Design review of the part built by this model. Coordinates are the model's own, in mm. Face numbers are marked on the shaded views. A direction names the side the tool comes from. Round coordinates to 2 decimals unless told otherwise and drop trailing zeros. Loops run counter-clockwise (first coordinate to the right, second up) from the corner with the lowest first, then second, coordinate; pieces in that order, holes last. Notation, with made-up numbers: M 15,70 L 60,70 A20 ccw 60,76 Z; hole C 41,39.25 d9. An arc over 180 degrees is marked long. Answer as CSV lines item,"result". Start each with the question number.
from build123d import *

# Parameters (mm, degrees)
F0_W      = 54
F0_H      = 56
F1_DEPTH  = 102
F2_W      = 90
F2_H      = 36
F3_DEPTH  = 59.1
F6_DEPTH  = 25
F7_W      = 18
F7_H      = 54
F8_DEPTH  = 8
F9_W      = 24
F9_H      = 54
F10_DEPTH = 8
F11_W     = 36
F11_H     = 54
F12_DEPTH = 8
F14_DEPTH = 12
F16_DEPTH = 25
F18_DEPTH = 42.4
F20_DEPTH = 25


with BuildPart() as f1:
    # F0 (on Right) → F1 (new body)
    with BuildSketch(Plane.YZ):
        with Locations((-4.050715, 4.935318)):
            Rectangle(F0_W, F0_H)
    extrude(amount=F1_DEPTH)

    # F2 (on face) → F3 (cut)
    with BuildSketch(Plane(origin=(0, 22.949285, 0), x_dir=(-1, 0, 0), z_dir=(0, 1, 0))):
        with Locations((-57, -5.064682)):
            Rectangle(F2_W, F2_H)
    extrude(amount=-F3_DEPTH, mode=Mode.SUBTRACT)

    # F5 (on face) → F6 (cut)
    with BuildSketch(Plane(origin=(0, 0, 0), x_dir=(0, -1, 0), z_dir=(-1, 0, 0))):
        Polygon((-2.864712, -16.520232), (11.135288, -16.520232), (20.040549, -5.717624), (11.135288, 5.084983), (-2.864712, 5.084983), (-11.769973, -5.717624), align=None)
    extrude(amount=-F6_DEPTH, mode=Mode.SUBTRACT)

    # F7 (on face) → F8 (cut)
    with BuildSketch(Plane.XY.offset(32.935318)):
        with Locations((9, -4.050715)):
            Rectangle(F7_W, F7_H)
    extrude(amount=-F8_DEPTH, mode=Mode.SUBTRACT)

    # F9 (on face) → F10 (cut)
    with BuildSketch(Plane.XY.offset(32.935318)):
        with Locations((42, -4.050715)):
            Rectangle(F9_W, F9_H)
    extrude(amount=-F10_DEPTH, mode=Mode.SUBTRACT)

    # F11 (on face) → F12 (cut)
    with BuildSketch(Plane.XY.offset(32.935318)):
        with Locations((84, -4.050715)):
            Rectangle(F11_W, F11_H)
    extrude(amount=-F12_DEPTH, mode=Mode.SUBTRACT)

    # F13 (on face) → F14 (cut)
    with BuildSketch(Plane.YZ.offset(66)):
        Polygon((16.72348, 32.935318), (-4.050715, 32.935318), (-4.050715, 24.935318), align=None)
    extrude(amount=-F14_DEPTH, mode=Mode.SUBTRACT)

    # F15 (on face) → F16 (cut)
    with BuildSketch(Plane.YZ.offset(66)):
        Polygon((-4.050715, 32.935318), (-24.917709, 32.935318), (-4.050715, 24.935318), align=None)
    extrude(amount=-F16_DEPTH, mode=Mode.SUBTRACT)

    # F17 (on face) → F18 (cut)
    with BuildSketch(Plane(origin=(0, 0, 0), x_dir=(0, -1, 0), z_dir=(-1, 0, 0))):
        Polygon((26.28649, 33.151057), (-16.84958, 33.434331), (4.061393, 24.936128), align=None)
    extrude(amount=-F18_DEPTH, mode=Mode.SUBTRACT)

    # F19 (on face) → F20 (cut)
    with BuildSketch(Plane.XY.offset(24.935318)):
        Polygon((96, -19.514816), (102, -16.050715), (102, 7.949285), (96, 11.413387), align=None)
    extrude(amount=-F20_DEPTH, mode=Mode.SUBTRACT)


solid = f1.part
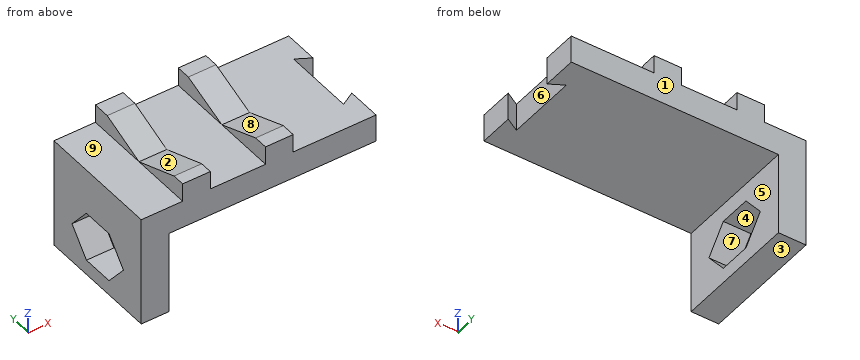
Item 1: Consider section C-C, the plane y = -2. Write out the cut boundary in (x, z), then the cut area to 3 significant figures.
Item 2: Consider section D-D, the plane z = 19. Write out the cut boundary in (x, y).
Item 3: Insertion check: pin 1 Ø14.5 at (x, y) = (8.5, -12.5) entering from +Z; pin 2 Ø6 at (y, z) = (-11.5, 16.5) entering from +X; pin 3 Ø6.5 at (y, z) = (-23, 28) entering from +X; pin 4 Ø4 at (x, y) = (26, 8.5) entering from -Z. Each pin has a flat end and moves straight along its axis. Give the tip position at first contact, or say it passes through.
Item 4: Consider section A-A, the plane z = 2.5. Write out the cut boundary in (x, y).
Item 5: Consider section B-B, the plane x = 28.5. Write out the cut boundary in (y, z).
Item 6: To check wall thickness, follow line 1 (X direction, y = -21, z = 26.5); line 2 (X direction, y = -9, z = 18.5); line 3 (Z direction, x = 10, y = 12.5). State the ranges of each line that lie inside material, in increasing order.
Item 7: The part is to be moulded in two halves that separate along Y. For the marked faces 1, 2, 3 and 4, say which applies: +Y half, -Y half, draft (parallel to the pull), parting line (faces both ways), or undercut.
Item 8: Tool access review of the marked faces 5, 6, 7, 8 and 9: name each direction out of +Z, -Z, +X, -X, +Y, -Y from which nothing blocks a thin tool from reaching the whole face with its end or side.
Found:
1,outline,"M 0,-23.06 L 12,-23.06 L 12,-16.52 L 0,-16.52 Z; M 0,5.08 L 12,5.08 L 12,12.94 L 96,12.94 L 96,24.94 L 66,24.94 L 66,25.73 L 54,25.73 L 54,24.94 L 30,24.94 L 30,25.77 L 18,25.77 L 18,24.94 L 0,24.94 Z"
1,area,"1,340 mm^2"
2,outline,"M 0,-31.05 L 102,-31.05 L 102,-16.05 L 96,-19.51 L 96,11.41 L 102,7.95 L 102,22.95 L 0,22.95 Z"
3,pin 1,"stops at z = 24.94"
3,pin 2,"stops at x = 96"
3,pin 3,"stops at x = 102"
3,pin 4,"stops at z = 12.94"
4,outline,"M 0,-31.05 L 12,-31.05 L 12,-13.27 L 0,-13.27 Z; M 0,5 L 12,5 L 12,22.95 L 0,22.95 Z"
5,outline,"M -31.05,12.94 L 22.95,12.94 L 22.95,32.94 L 15.62,32.94 L -4.06,24.94 L -25.7,32.94 L -31.05,32.94 Z"
6,line 1,"x = 18 to 30, 54 to 66"
6,line 2,"x = 0 to 96"
6,line 3,"z = -23.06 to 24.94"
7,face 1,"+Y half"
7,face 2,"undercut"
7,face 3,"draft"
7,face 4,"undercut"
8,face 5,"-Z, +X, +Y, -Y"
8,face 6,"+Z, -Z"
8,face 7,"+X, -X"
8,face 8,"+Z, +X, -X"
8,face 9,"+Z, -X, +Y, -Y"
